Geometry: final body of the model. Coordinates: model frame, mm. A direction names the side the tool comes from. Round coordinates to 2 decimals unless told otherwise and drop trailing zeros. Loops run counter-clockwise (first coordinate to the right, second up) from the corner with the lowest first, then second, coordinate; pieces in that order, holes last. Notation, with made-up numbers: (41.5, 73) -> (54.5, 73) arc R34 ccw to (54.5, 110) -> close; hole circle Ø3 at (27, 33.5). An arc over 180 degrees is marked (long way). Answer in a Markdown table with one row per item.
```python
from build123d import *

# Parameters (mm, degrees)
BOSS_EXTRUDE1_DEPTH     = 39.35
CUT_EXTRUDE2_DEPTH      = 33.73
CUT_EXTRUDE2_DEPTH_BACK = 3
SKETCH3_R               = 5.1
CUT_EXTRUDE3_DEPTH      = 33.73
CUT_EXTRUDE4_DEPTH      = 87.647311883
CUT_EXTRUDE4_DEPTH_BACK = 87.647311883
SKETCH3_5_R             = 3.1
SKETCH3_5_R_2           = 10.1
SKETCH3_5_R_3           = 1.6
SKETCH3_5_W             = 20.675
SKETCH3_5_H             = 20.2
SKETCH3_5_W_2           = 5.027537917
SKETCH3_5_H_2           = 3.2
SKETCH3_5_W_3           = 5.03
SKETCH3_6_R             = 1.6
CUT_EXTRUDE5_DEPTH      = 87.647311883
SKETCH4_W               = 77.35
SKETCH4_H               = 38.73
BOSS_EXTRUDE2_DEPTH     = 4
SKETCH5_W               = 77.35
SKETCH5_H               = 38.73
BOSS_EXTRUDE3_DEPTH     = 4
CUT_EXTRUDE6_DEPTH      = 92.909209967
CUT_EXTRUDE6_DEPTH_BACK = 92.909209967
CUT_EXTRUDE7_DEPTH      = 2.5
CHAMFER1_SIZE           = 14
CHAMFER1_SIZE_2         = 24.248711306


with BuildPart() as part:
    # Sketch1 → Boss-Extrude1 (new body)
    with BuildSketch(Plane.XY):
        Polygon((-68.943174111, 38.106680783), (-32.943174111, 38.106680783), (-32.943174111, 3.376680783), (8.406825889, 3.376680783), (8.406825889, -0.623319217), (-68.943174111, -0.623319217), (-68.943174111, 3.376680783), (-36.943174111, 3.376680783), (-36.943174111, 34.106680783), (-68.943174111, 34.106680783), align=None)
    extrude(amount=BOSS_EXTRUDE1_DEPTH)

    # Sketch3 → Cut-Extrude2 (cut, two sides: drawn at the far end of the back side and taken through both)
    with BuildSketch(Plane(origin=(0, 3.376680783, 0), x_dir=(1, 0, 0), z_dir=(0, 1, 0)).offset(-CUT_EXTRUDE2_DEPTH_BACK)):
        with Locations(Location((-52.943174111, -19.675, 0), (0, 0, 90))):
            Circle(SKETCH3_R)
    extrude(amount=CUT_EXTRUDE2_DEPTH + CUT_EXTRUDE2_DEPTH_BACK, mode=Mode.SUBTRACT)

    # Sketch3<4> → Cut-Extrude3 (cut)
    with BuildSketch(Plane(origin=(0, 3.376680783, 0), x_dir=(1, 0, 0), z_dir=(0, 1, 0))):
        with BuildLine():
            Line((-47.58710279, -20.925), (-45.294644841, -20.925))
            Line((-45.294644841, -20.925), (-45.294644841, -18.425))
            Line((-45.294644841, -18.425), (-47.58710279, -18.425))
            ThreePointArc((-47.58710279, -18.425), (-47.479274758, -19.045870549), (-47.443174111, -19.675))
            ThreePointArc((-47.443174111, -19.675), (-47.479274758, -20.304129451), (-47.58710279, -20.925))
        make_face()
        with BuildLine():
            Line((-60.591703381, -18.425), (-60.591703381, -20.925))
            Line((-60.591703381, -20.925), (-58.299245432, -20.925))
            ThreePointArc((-58.299245432, -20.925), (-58.443174111, -19.675), (-58.299245432, -18.425))
            Line((-58.299245432, -18.425), (-60.591703381, -18.425))
        make_face()
    extrude(amount=CUT_EXTRUDE3_DEPTH, mode=Mode.SUBTRACT)

    # Sketch3<5> → Cut-Extrude4 (cut, two sides: drawn at the far end of the back side and taken through both)
    with BuildSketch(Plane(origin=(0, 3.376680783, 0), x_dir=(1, 0, 0), z_dir=(0, 1, 0)).offset(-CUT_EXTRUDE4_DEPTH_BACK)):
        with Locations(Location((-52.943174111, -19.675, 0), (0, 0, 270))):
            Circle(SKETCH3_5_R)
        with Locations((-12.268174111, -19.675)):
            Circle(SKETCH3_5_R_2)
        with Locations((-4.768174111, -32.665381057)):
            Circle(SKETCH3_5_R_3)
        with Locations((-4.768174111, -6.684618943)):
            Circle(SKETCH3_5_R_3)
        with Locations((-27.268174111, -19.675)):
            Circle(SKETCH3_5_R_3)
        with Locations((0.261825889, -32.665381057)):
            Circle(SKETCH3_5_R_3)
        with Locations((0.261825889, -6.684618943)):
            Circle(SKETCH3_5_R_3)
        with Locations((-1.930674111, -19.675)):
            Rectangle(SKETCH3_5_W, SKETCH3_5_H)
        with Locations((-24.754405152, -19.675)):
            Rectangle(SKETCH3_5_W_2, SKETCH3_5_H_2)
        with Locations((-2.253174111, -32.665381057)):
            Rectangle(SKETCH3_5_W_3, SKETCH3_5_H_2)
        with Locations((-2.253174111, -6.684618943)):
            Rectangle(SKETCH3_5_W_3, SKETCH3_5_H_2)
    extrude(amount=CUT_EXTRUDE4_DEPTH + CUT_EXTRUDE4_DEPTH_BACK, mode=Mode.SUBTRACT)

    # Sketch3<6> → Cut-Extrude5 (cut, through all)
    with BuildSketch(Plane(origin=(0, 3.376680783, 0), x_dir=(1, 0, 0), z_dir=(0, 1, 0))):
        with Locations(Location((-52.943174111, -34.675, 0), (0, 0, 180))):
            Circle(SKETCH3_6_R)
        with Locations(Location((-65.933555168, -27.175, 0), (0, 0, 180))):
            Circle(SKETCH3_6_R)
        with Locations(Location((-65.933555168, -12.175, 0), (0, 0, 180))):
            Circle(SKETCH3_6_R)
        with Locations(Location((-52.943174111, -4.675, 0), (0, 0, 180))):
            Circle(SKETCH3_6_R)
        with Locations(Location((-39.952793054, -12.175, 0), (0, 0, 180))):
            Circle(SKETCH3_6_R)
        with Locations(Location((-39.952793054, -27.175, 0), (0, 0, 180))):
            Circle(SKETCH3_6_R)
    extrude(amount=CUT_EXTRUDE5_DEPTH, mode=Mode.SUBTRACT)

    # Sketch4 → Boss-Extrude2 (add)
    with BuildSketch(Plane.XY.offset(39.35)):
        with Locations((-30.268174111, 18.741680783)):
            Rectangle(SKETCH4_W, SKETCH4_H)
    extrude(amount=BOSS_EXTRUDE2_DEPTH)

    # Sketch5 → Boss-Extrude3 (add)
    with BuildSketch(Plane(origin=(0, 0, 0), x_dir=(-1, 0, 0), z_dir=(0, 0, -1))):
        with Locations((30.268174111, 18.741680783)):
            Rectangle(SKETCH5_W, SKETCH5_H)
    extrude(amount=BOSS_EXTRUDE3_DEPTH)

    # Sketch6 → Cut-Extrude6 (cut, two sides: drawn at the far end of the back side and taken through both)
    with BuildSketch(Plane.XY.offset(43.35).offset(-CUT_EXTRUDE6_DEPTH_BACK)):
        Polygon((-32.943174111, 38.106680783), (5.861825889, 3.376680783), (5.861825889, -0.623319217), (8.406825889, -0.623319217), (8.406825889, 38.106680783), align=None)
    extrude(amount=CUT_EXTRUDE6_DEPTH + CUT_EXTRUDE6_DEPTH_BACK, mode=Mode.SUBTRACT)

    # Sketch8 → Cut-Extrude7 (cut)
    with BuildSketch(Plane.XZ.offset(-34.106680783)):
        Polygon((-65.933555168, 15.408161507), (-68.733555168, 13.791580754), (-68.733555168, 10.558419246), (-65.933555168, 8.941838493), (-63.133555168, 10.558419246), (-63.133555168, 13.791580754), align=None)
        Polygon((-65.933555168, 30.408161507), (-68.733555168, 28.791580754), (-68.733555168, 25.558419246), (-65.933555168, 23.941838493), (-63.133555168, 25.558419246), (-63.133555168, 28.791580754), align=None)
        Polygon((-52.943174111, 1.441838493), (-50.143174111, 3.058419246), (-50.143174111, 6.291580754), (-52.943174111, 7.908161507), (-55.743174111, 6.291580754), (-55.743174111, 3.058419246), align=None)
        Polygon((-39.952793054, 8.941838493), (-37.152793054, 10.558419246), (-37.152793054, 13.791580754), (-39.952793054, 15.408161507), (-42.752793054, 13.791580754), (-42.752793054, 10.558419246), align=None)
        Polygon((-39.952793054, 23.941838493), (-37.152793054, 25.558419246), (-37.152793054, 28.791580754), (-39.952793054, 30.408161507), (-42.752793054, 28.791580754), (-42.752793054, 25.558419246), align=None)
        Polygon((-52.943174111, 37.908161507), (-55.743174111, 36.291580754), (-55.743174111, 33.058419246), (-52.943174111, 31.441838493), (-50.143174111, 33.058419246), (-50.143174111, 36.291580754), align=None)
    extrude(amount=-CUT_EXTRUDE7_DEPTH, mode=Mode.SUBTRACT)

    # Chamfer1
    # the kernel refuses this chamfer: 24.248711306, 14 mm, written as the material it takes off along each edge
    with BuildSketch(Plane(origin=(-68.943174111, -63.356814805, 43.35), x_dir=(-0.05789386240267122, 0, -0.9983227437537925), z_dir=(0, 1, 0))) as chamfer1_piece_1:
        Polygon((CHAMFER1_SIZE * 0.998322743754, -CHAMFER1_SIZE * 0.0578938624027), (-CHAMFER1_SIZE_2 * 0.0578938624026, -CHAMFER1_SIZE_2 * 0.998322743752), (0, 0), align=None)
    extrude(amount=164.196991176, mode=Mode.SUBTRACT)
    with BuildSketch(Plane(origin=(-68.943174111, -63.356814805, -4), x_dir=(-0.05789386240267123, 0, 0.9983227437537925), z_dir=(0, 1, 0))) as chamfer1_piece_2:
        Polygon((CHAMFER1_SIZE * 0.998322743754, CHAMFER1_SIZE * 0.0578938624027), (-CHAMFER1_SIZE_2 * 0.0578938624026, CHAMFER1_SIZE_2 * 0.998322743752), (0, 0), align=None)
    extrude(amount=164.196991176, mode=Mode.SUBTRACT)


solid = part.part
```
Item 1: First-contact query: P1, Ø4.5, axis at x = -47.5, y = 20.5, coming from the -Z side; P2, Ø19.5, axis at x = -13.5, z = 20.5, coming from the +Y side; P3, Ø1, axis at y = 5.5, z = 31.5, coming from the +X side. Flat tips, straight axial feed; report the tip coordinate or a pass-through.
Ans:
| item | result |
|---|---|
| P1 | z = -3.68 |
| P2 | y = 3.38 |
| P3 | x = -32.94 |
Item 2: Section query B-B, the plane y = 22. Output: boundary loops of the cut face in (x, z), and give its area (3 significant figures).
Ans:
| item | result |
|---|---|
| outline | (-51.62, 0) -> (-44.69, -4) -> (-14.95, -4) -> (-14.95, 0) -> (-32.94, 0) -> (-32.94, 39.35) -> (-14.95, 39.35) -> (-14.95, 43.35) -> (-44.69, 43.35) -> (-51.62, 39.35) -> (-36.94, 39.35) -> (-36.94, 0) -> close |
| area | 423 mm2 |
Item 3: Section query A-A, the plane y = 12. Output: boundary loops of the cut face in (x, z).
Ans:
| item | result |
|---|---|
| outline | (-51.62, 0) -> (-44.69, -4) -> (-3.77, -4) -> (-3.77, 0) -> (-32.94, 0) -> (-32.94, 39.35) -> (-3.77, 39.35) -> (-3.77, 43.35) -> (-44.69, 43.35) -> (-51.62, 39.35) -> (-36.94, 39.35) -> (-36.94, 0) -> close |
Item 4: Mould query, pull axis X, two halves, no side actions, for faces 5 (the flat face through (-48.906, 18.471, -1.569)), 6 (the flat face through (-38.57, 35.34, 24.74)), 7 (the flat face through (-22, 3.377, 24)), 8 (the cylindrical face through (-18.74, 1.35, 11.92)). Classes: released by +X, released by -X, zero draft, split by the parting line, or undercut.
Ans:
| item | result |
|---|---|
| face 5 | released by -X |
| face 6 | undercut |
| face 7 | zero draft |
| face 8 | released by +X |
Item 5: Set-up query: faces 1 (the flat face through (-36.943, 19, 19)), 2 (the cylindrical face through (-53.681, 37.346, 33.256)), 3 (the flat face through (-55.743, 35, 5)), 4 (the flat face through (-2, 1, 31.065)). Return all of +Z, -Z, +X, -X, +Y, -Y with unobstructed straight access to the full face (end or side cutting, diameter ignored); none if empty.
Ans:
| item | result |
|---|---|
| face 1 | -X |
| face 2 | +Y |
| face 3 | none |
| face 4 | +Y, -Y |
Item 6: Ray query, L1, parallel to Z at x = -15.5, y = 5; L2, parallel to Y at x = -46.5, z = 24.5; L3, parallel to X at y = 25, z = 17. Return the intervals inside material, ascending.
Ans:
| item | result |
|---|---|
| L1 | -4 to 0, 39.35 to 43.35 |
| L2 | -0.62 to 3.38, 34.11 to 38.11 |
| L3 | -36.94 to -32.94 |
